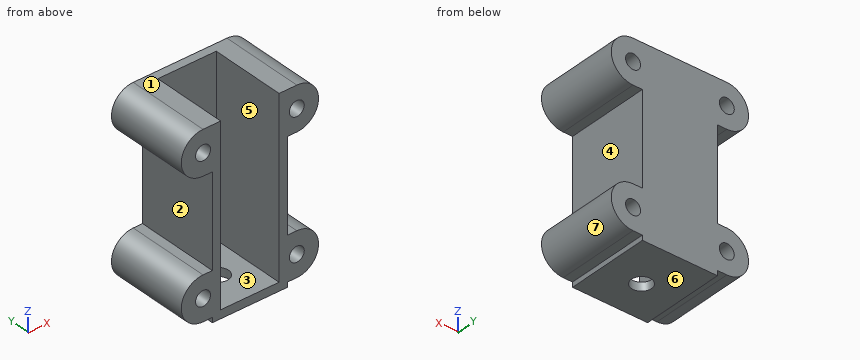
Autodesk Inventor part; units mm, degrees
ref_plane "Work Plane1" through (7.1438, 0, 33.3375) normal (-1, 0, 0) x (0, 0, -1)
ref_plane "YZ Plane" through (0, 0, 0) normal (1, 0, 0) x (0, 1, 0)
ref_plane "XZ Plane" through (0, 0, 0) normal (0, 1, 0) x (-1, 0, 0)
sketch "Sketch1" plane through (0, 0, 0) normal (0, 0, 1) x (1, 0, 0)
  line L0 (0, 0) -> (1.5875, 0)
  line L1 (1.5875, 0) -> (1.5875, 14.2875)
  line L2 (1.5875, 14.2875) -> (12.7, 14.2875)
  line L3 (12.7, 14.2875) -> (12.7, 0)
  line L4 (12.7, 0) -> (14.2875, 0)
  line L5 (14.2875, 0) -> (14.2875, 15.875)
  line L6 (14.2875, 15.875) -> (0, 15.875)
  line L7 (0, 15.875) -> (0, 0)
  dimension "d1" = 11.1125
  dimension "wallThickness" = 1.5875
  dimension "d4" = 1.5875
  dimension "d5" = 1.5875
  dimension "d6" = 14.2875
  dimension "outerWidth" = 14.2875
extrude "Extrusion1" add sketch "Sketch1" along normal blind 33.3375
sketch "Sketch2" plane through (0, 0, 0) normal (0, 0, -1) x (-1, 0, 0)
  line L0 (0, 15.875) -> (0, 0)
  line L1 (-14.2875, 15.875) -> (0, 15.875)
  line L2 (-14.2875, 0) -> (-14.2875, 15.875)
  line L3 (-14.2875, 0) -> (0, 0)
  line L4 (-12.7, 14.2875) -> (-12.7, 0)
  circle A0 centre (-7.1437, 7.1437) radius 1.905
  dimension "d11" = 3.81
  dimension "d12" = 7.1437
  dimension "d13" = 5.5563
extrude "Extrusion3" add sketch "Sketch2" along normal blind 1.5875
sketch "Sketch3" plane through (0, 15.875, 33.3375) normal (0, 1, 0) x (1, 0, 0)
  line L0 (0, 34.925) -> (0, 0)
  circle A0 centre (-1.778, 4.1406) radius 1.4224
  line L1 (0, 0) -> (-1.778, 0)
  line L2 (0, 8.2812) -> (-1.778, 8.2812)
  arc A1 (-1.778, 8.2812) -> (-1.778, 0) centre (-1.778, 4.1406) ccw
  line L3 (0, 0) -> (14.2875, 0)
  point P0 (0, 33.3375)
  dimension "screwOuterDiameter" = 8.2812
  dimension "d24" = 4.1406
  dimension "d25" = 0
  dimension "screwHoleOffsetFromSide" = 1.778
  dimension "screwHoleDiameter" = 2.8448
extrude "Extrusion4" add sketch "Sketch3" against normal blind 15.875
pattern_linear "Rectangular Pattern1" count 2 spacing 25.7175 along (0, 0, -1) of "Extrusion4"
ref_plane "Work Plane1" through (7.1438, 0, 33.3375) normal (-1, 0, 0) x (0, 0, -1)
mirror "Mirror1" about plane through (7.1438, 0, 33.3375) normal (-1, 0, 0) of "Extrusion4", "Rectangular Pattern1"
equation "\"d1\" = plungerWidth + plungerTolerance"
equation "\"d4\" = wallThickness"
equation "\"d5\" = wallThickness"
equation "\"d6\" = plungerHeight + plungerTolerance"
equation "\"outerLength\" = plungerLength + springLength"
equation "\"d12\" = 0.5 * d6"
equation "\"d13\" = 0.5 * d1"
equation "\"d14\" = wallThickness"
equation "\"d24\" = 0.5 * screwOuterDiameter"
equation "\"d28\" = wallThickness + plungerHeight + plungerTolerance"
properties part number "BatteryLatch-Outer"
CAD build for the part. Positions are in the model's coordinates, mm. Face numbers are marked on the shaded views. A direction names the side the tool comes from. Round coordinates to 2 decimals unless told otherwise and drop trailing zeros. Write each loop counter-clockwise with the first axis right and the second up, starting at its lowest first coordinate (ties: lowest second). Pieces come first, ordered by that corner, then holes.
(1) Slice it at C-C, the plane x = 18.75. Write the cut outline in (y, z) (3 decimals).
(2) 3-axis set-ups, long thin cutter, end or side, ignore diameter. For the marked faces 1, 2, 3 and 4: which of +Z, -Z, +X, -X, +Y, -Y reach the whole face in a straight line?
(3) Slice it at B-B, the plane z = 21.5. Write the cut outline in (x, y) (1 decimal), and give its area (3 significant figures).
(4) Slice it at D-D, the plane y = 11.5. Write the cut outline in (x, z).
(5) Slice it at A-A, the plane y = 8.5. Write the cut outline in (x, z).
(6) Mould opens along X. For the marked faces 5, 6 and 7 say: pulls with the +X half, pulls with the -X half, needs draft (parallel to the pull), parting line crosses it, or undercut.
(7) Probe line 1 along X through (y, z) = (11.75, 14); line 2 along X through (y, z) = (15, 4); line 3 along Z through (x, y) = (6.5, 9.5). List the from-to ranges inside material, lowest first.
(8) Drop flat-ended pins along their axis: P1, Ø3.5, axis at x = 7.14, y = 7.14, coming from the +Z side; P2, Ø7, axis at y = 8, z = 20.5, coming from the -X side; P3, Ø5.5, axis at x = 9, z = 24, coming from the -Y side; P4, Ø4.5, axis at x = 16.07, z = 3.48, coming from the -Y side. Give the stop position or say it passes through.
From the geometry:
1. outline: (0, 0.327) - (15.875, 0.327) - (15.875, 6.632) - (0, 6.632) - close; (0, 26.044) - (15.875, 26.044) - (15.875, 32.349) - (0, 32.349) - close
2. face 1: +Z, +X, -X, +Y, -Y
2. face 2: -X, +Y, -Y
2. face 3: +Z, -Y
2. face 4: +X, +Y, -Y
3. outline: (0, 0) - (1.6, 0) - (1.6, 14.3) - (12.7, 14.3) - (12.7, 0) - (14.3, 0) - (14.3, 15.9) - (0, 15.9) - close
3. area: 68.0 mm2
4. outline: (-1.78, -0.66) - (0, -0.66) - (0, -1.59) - (14.29, -1.59) - (14.29, -0.66) - (16.07, -0.66) arc R4.14 ccw to (16.07, 7.62) - (14.29, 7.62) - (14.29, 25.06) - (16.07, 25.06) arc R4.14 ccw to (16.07, 33.34) - (12.7, 33.34) - (12.7, 0) - (1.59, 0) - (1.59, 33.34) - (-1.78, 33.34) arc R4.14 ccw to (-1.78, 25.06) - (0, 25.06) - (0, 7.62) - (-1.78, 7.62) arc R4.14 ccw to start; hole circle Ø2.84 at (-1.78, 3.48); hole circle Ø2.84 at (-1.78, 29.2); hole circle Ø2.84 at (16.07, 3.48); hole circle Ø2.84 at (16.07, 29.2)
5. outline: (-1.78, -0.66) - (0, -0.66) - (0, -1.59) - (5.81, -1.59) - (5.81, 0) - (1.59, 0) - (1.59, 33.34) - (-1.78, 33.34) arc R4.14 ccw to (-1.78, 25.06) - (0, 25.06) - (0, 7.62) - (-1.78, 7.62) arc R4.14 ccw to start; (8.48, -1.59) - (14.29, -1.59) - (14.29, -0.66) - (16.07, -0.66) arc R4.14 ccw to (16.07, 7.62) - (14.29, 7.62) - (14.29, 25.06) - (16.07, 25.06) arc R4.14 ccw to (16.07, 33.34) - (12.7, 33.34) - (12.7, 0) - (8.48, 0) - close; hole circle Ø2.84 at (-1.78, 3.48); hole circle Ø2.84 at (-1.78, 29.2); hole circle Ø2.84 at (16.07, 3.48); hole circle Ø2.84 at (16.07, 29.2)
6. face 5: undercut
6. face 6: needs draft
6. face 7: pulls with the +X half
7. line 1: x = 0 to 1.59, 12.7 to 14.29
7. line 2: x = -5.89 to -3.1, -0.45 to 14.74, 17.39 to 20.17
7. line 3: z = -1.59 to 0
8. P1: passes through
8. P2: stops at x = 0
8. P3: stops at y = 14.29
8. P4: stops at y = 0
